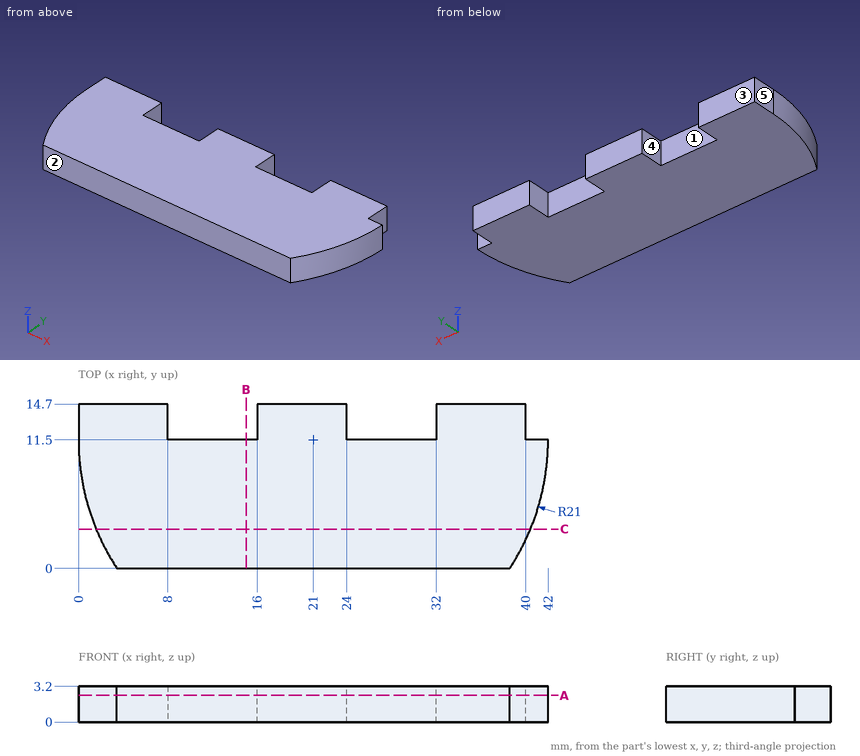
Design review of the part shown in the three views and the two pictorial views. Dimensions are in mm from the part's minimum x, y and z. A direction names the side the tool comes from. Give positions to 0.01 mm unless a question says otherwise; leave off trailing zeros. Loops run counter-clockwise (first coordinate to the right, second up) from the corner with the lowest first, then second, coordinate; pieces in that order, holes last. Notation, with made-up numbers: (37.5, 15.25) -> (42.5, 15.25) arc R22 cw to (42.5, 45.25) -> close; hole circle Ø4 at (2.25, -39). An arc over 180 degrees is marked (long way). Put each result on its own line as item: value. Start each with the question number.
1. We need section C-C on y = 3.5. State the section outline as (x, z) points.
2. We need section B-B on x = 15. State the section outline as (y, z) points, then the cut area to 3 significant figures.
3. For the marked faces 1 and 2, list the 3-axis set-ups (+Z, -Z, +X, -X, +Y, -Y) from which the entire face can be reached by the end or side of a thin tool; tool diameter is ignored.
4. We need section A-A on z = 2.4. State the section outline as (x, y) points.
5. Clearance check with a flat-ended pin moving along its axis: P1, Ø1.6, axis at y = 13, z = 1, coming from the +X side. State where the tip first meets the part, or that it passes through.
6. Wall thickness on probe 1 along X at (y, z) = (12.5, 2.8); probe 2 along Y at (x, z) = (31, 1.05); probe 3 along X at (y, z) = (2.75, 3): over which ranges is each line inside the solid? List them lowest first.
7. Mouldability with a two-part tool opening along X and no side actions: class the marked faces 3, 4 and 5 as released by +X, released by -X, zero draft, split by the parting line, or undercut.
Determined:
1. outline: (1.58, 0) -> (40.42, 0) -> (40.42, 3.2) -> (1.58, 3.2) -> close
2. outline: (0, 0) -> (11.5, 0) -> (11.5, 3.2) -> (0, 3.2) -> close
2. area: 36.8 mm^2
3. face 1: +Z, -Z, +Y
3. face 2: +Z, -Z, +X, -X, -Y
4. outline: (0, 11.5) arc R21 ccw to (3.43, 0) -> (38.57, 0) arc R21 ccw to (42, 11.5) -> (40, 11.5) -> (40, 14.7) -> (32, 14.7) -> (32, 11.5) -> (24, 11.5) -> (24, 14.7) -> (16, 14.7) -> (16, 11.5) -> (8, 11.5) -> (8, 14.7) -> (0, 14.7) -> close
5. P1: x = 40
6. probe 1: 0 to 8, 16 to 24, 32 to 40
6. probe 2: 0 to 11.5
6. probe 3: 1.91 to 40.09
7. face 3: zero draft
7. face 4: undercut
7. face 5: released by -X
